Geometry: final body of the model. Coordinates: model frame, mm. A direction names the side the tool comes from. Give positions to 0.01 mm unless a question says otherwise; leave off trailing zeros. Order: outer loops, then holes, each group sorted by start corner. A loop starts at its lowest first (then second) coordinate and runs counter-clockwise, first axis right, second up. Notation, with made-up numbers: (20, 54.25) - (30, 54.25) arc R26 cw to (30, 84.25) - close; hole circle Ø8 at (59, 43). An arc over 180 degrees is marked (long way). One line per item, written item: value.
```python
from build123d import *

# Parameters (mm, degrees)
SKETCH1_R           = 8
BOSS_EXTRUDE1_DEPTH = 2
SKETCH2_R           = 3.75
BOSS_EXTRUDE2_DEPTH = 38
RIB2_REACH          = 43.569
SKETCH3_WALL_W      = 87.966865888
SKETCH3_WALL_H      = 2
SKETCH5_W           = 2
SKETCH5_H           = 0.73
FILLET1_R           = 0.5
CHAMFER1_SIZE       = 1.5


with BuildPart() as part:
    # Sketch1 → Boss-Extrude1 (new body)
    with BuildSketch(Plane(origin=(0, 0, 0), x_dir=(1, 0, 0), z_dir=(0, 1, 0))):
        with Locations(Location((0, 0, 0), (0, 0, 270))):
            Circle(SKETCH1_R)
    extrude(amount=-BOSS_EXTRUDE1_DEPTH)

    # Sketch2 → Boss-Extrude2 (add)
    with BuildSketch(Plane.XZ.offset(2)):
        with Locations(Location((0, 0, 0), (0, 0, 270))):
            Circle(SKETCH2_R)
    extrude(amount=BOSS_EXTRUDE2_DEPTH)

    # Sketch3 wall → Rib2 (add, up to next)
    with BuildSketch(Plane(origin=(4.75, -3, 0), x_dir=(-0.707106781187, -0.707106781187, 0), z_dir=(0.707106781187, -0.707106781187, 0)), mode=Mode.PRIVATE) as rib2_sk1:
        Rectangle(SKETCH3_WALL_W, SKETCH3_WALL_H)
    rib2_tool1 = extrude(rib2_sk1.sketch, amount=-RIB2_REACH, mode=Mode.PRIVATE) - part.part
    add(rib2_tool1.solids().sort_by_distance((4.75, -3, 0))[0])

    # Sketch5 → Cut-Revolve1 (revolve, cut)
    with BuildSketch(Plane(origin=(0, 0, 0), x_dir=(0, 0, -1), z_dir=(1, 0, 0))):
        with Locations((4.2, -37.365)):
            Rectangle(SKETCH5_W, SKETCH5_H)
    revolve(axis=Axis((0, -40, 0), (0, 1, 0)), mode=Mode.SUBTRACT)

    # Fillet1
    fillet1_edges = [part.edges().sort_by_distance(p)[0] for p in [
        (0, 0, -8),
        (0, -2, -8),
    ]]
    fillet(fillet1_edges, radius=FILLET1_R)

    # Chamfer1
    chamfer1_edges = [part.edges().sort_by_distance(p)[0] for p in [
        (0, -40, 3.75),
    ]]
    chamfer(chamfer1_edges, length=CHAMFER1_SIZE)


solid = part.part
```
1) Mould query, pull axis Y, two halves, no side actions, for faces 4 (the face through (0, 0, 0)), 5 (the face through (-3, -2, 3)), 6 (the face through (4, -3, 1)), 7 (the face through (1.947, -37.36, 2.539)). Classes: released by +Y, released by -Y, zero draft, split by the parting line, or undercut.
Answers below:
face 4: released by +Y
face 5: released by -Y
face 6: zero draft
face 7: undercut
2) Material intervals for line 1 along Y through (x, z) = (-6, -0.75); line 2 along X through (y, z) = (-14, 3); line 3 along Z through (x, y) = (-2.25, -25), sorted ascending.
Answers below:
line 1: -2 to 0
line 2: -2.25 to 2.25
line 3: -3 to 3
3) Section A-A, the plane z = 0. Return loops of the section in (x, y).
Answers below:
outline: (-8, -1.5) arc R0.5 ccw to (-7.5, -2) - (-3.75, -2) - (-3.75, -37) - (-3.2, -37) - (-3.2, -37.73) - (-3.75, -37.73) - (-3.75, -38.5) - (-2.25, -40) - (2.25, -40) - (3.75, -38.5) - (3.75, -37.73) - (3.2, -37.73) - (3.2, -37) - (3.75, -37) - (3.75, -4) - (5.75, -2) - (7.5, -2) arc R0.5 ccw to (8, -1.5) - (8, -0.5) arc R0.5 ccw to (7.5, 0) - (-7.5, 0) arc R0.5 ccw to (-8, -0.5) - close
4) First-contact query: pin 1 (1.1 mm diameter, centred on x = 5, y = -3, fed in from +Z); pin 2 (6 mm diameter, centred on x = -3.5, z = 3.5, fed in from -Y); pin 3 (6 mm diameter, centred on x = 4.5, z = 4.5, fed in from -Y); pin 4 (8 mm diameter, centred on x = 5.5, z = 3.5, fed in from -Y). Flat tips, straight axial feed; report the tip coordinate or a pass-through.
Answers below:
pin 1: z = 1
pin 2: y = -40
pin 3: y = -38.89
pin 4: y = -39.73
5) Set-up query: faces 1 (the face through (-7.81, -0.99, -1.73)), 2 (the face through (4, -3, -1)), 3 (the face through (0.165, -38.11, 3.746)). Return all of +Z, -Z, +X, -X, +Y, -Y with unobstructed straight access to the full face (end or side cutting, diameter ignored); none if empty.
Answers below:
face 1: +Y, -Y
face 2: -Z, +X, -Y
face 3: -Y
6) Section B-B, the plane x = 0. Return loops of the section in (y, z), then the cut area to 3 significant figures.
Answers below:
outline: (-40, -2.25) - (-38.5, -3.75) - (-37.73, -3.75) - (-37.73, -3.2) - (-37, -3.2) - (-37, -3.75) - (-2, -3.75) - (-2, -7.5) arc R0.5 ccw to (-1.5, -8) - (-0.5, -8) arc R0.5 ccw to (0, -7.5) - (0, 7.5) arc R0.5 ccw to (-0.5, 8) - (-1.5, 8) arc R0.5 ccw to (-2, 7.5) - (-2, 3.75) - (-37, 3.75) - (-37, 3.2) - (-37.73, 3.2) - (-37.73, 3.75) - (-38.5, 3.75) - (-40, 2.25) - close
area: 314 mm^2
7) Section C-C, the plane y = -17.5. Return loops of the section in (x, z), then the cut area to 3 significant figures.
Answers below:
outline: circle Ø7.5 at (0, 0)
area: 44.2 mm^2
